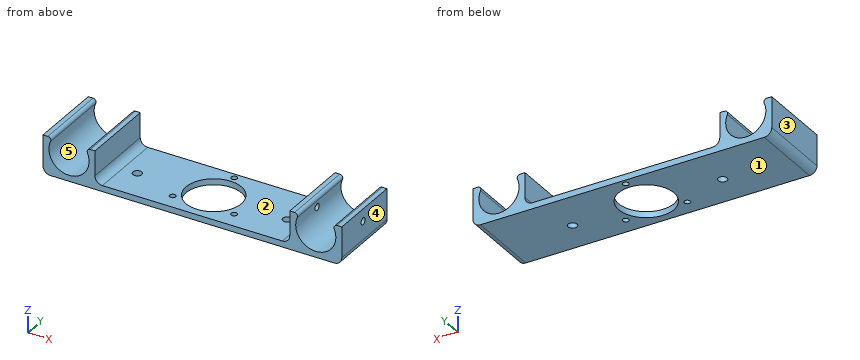
```python
from build123d import *

# Parameters (mm, degrees)
BOSS_EXTRUDE2_START = -1
SKETCH1_R           = 13.45
BOSS_EXTRUDE2_DEPTH = 53
FILLET1_R           = 3
FILLET2_R           = 5
SKETCH9_R           = 2.25
CUT_EXTRUDE2_DEPTH  = 175.062632406
CUT_EXTRUDE4_DEPTH  = 61
FILLET3_R           = 2
SKETCH12_R          = 18.5
SKETCH12_R_2        = 2
CUT_EXTRUDE5_DEPTH  = 61
SKETCH13_R          = 3
CUT_EXTRUDE8_DEPTH  = 41
SKETCH14_W          = 211.811280225
SKETCH14_H          = 13.838629025
CUT_EXTRUDE10_DEPTH = 41


with BuildPart() as part:
    # Sketch1 → Boss-Extrude2 (new body)
    with BuildSketch(Plane(origin=(0, 0, 0), x_dir=(1, 0, 0), z_dir=(0, 1, 0)).offset(BOSS_EXTRUDE2_START)):
        Polygon((-17.4, 17.4), (17.4, 17.4), (17.4, -17.4), (-17.4, -17.4), (-17.4, 13.4), (-82.6, 13.4), (-82.6, 17.4), align=None)
        with Locations(Location((0, 0, 0), (0, 0, 270))):
            Circle(SKETCH1_R, mode=Mode.SUBTRACT)
    boss_extrude2 = extrude(amount=BOSS_EXTRUDE2_DEPTH)

    # Mirror2: Boss-Extrude2 across plane
    add(boss_extrude2.mirror(Plane(origin=(-82.6, -1, -17.4), x_dir=(0, 0, 1), z_dir=(-1, 0, 0))))

    # Fillet1
    fillet1_edges = [part.edges().sort_by_distance(p)[0] for p in [
        (17.4, 25.5, 17.4),
        (-17.4, 25.5, 17.4),
        (-182.6, 25.5, 17.4),
        (-147.8, 25.5, 17.4),
    ]]
    fillet(fillet1_edges, radius=FILLET1_R)

    # Fillet2
    fillet2_edges = [part.edges().sort_by_distance(p)[0] for p in [
        (-17.4, 25.5, -13.4),
        (17.4, 25.5, -17.4),
        (-182.6, 25.5, -17.4),
        (-147.8, 25.5, -13.4),
    ]]
    fillet(fillet2_edges, radius=FILLET2_R)

    # Sketch9 → Cut-Extrude2 (cut, through all)
    with BuildSketch(Plane.ZY.offset(17.4)):
        with Locations((0, 25.5)):
            Circle(SKETCH9_R)
    extrude(amount=-CUT_EXTRUDE2_DEPTH, mode=Mode.SUBTRACT)

    # Sketch11 → Cut-Extrude4 (cut)
    with BuildSketch(Plane.XZ.offset(1)):
        Polygon((17.4, 11.356288415), (17.4, 18.363602968), (-17.4, 18.363602968), (-17.4, 11.356288415), (-17.4, 8.165104504), (-10.6880105, 8.165104504), (10.6880105, 8.165104504), (17.4, 8.165104504), align=None)
        Polygon((-182.6, 11.356288415), (-182.6, 18.363602968), (-147.8, 18.363602968), (-147.8, 11.356288415), (-147.8, 8.165104504), (-154.5119895, 8.165104504), (-175.8880105, 8.165104504), (-182.6, 8.165104504), align=None)
    extrude(amount=-CUT_EXTRUDE4_DEPTH, mode=Mode.SUBTRACT)

    # Fillet3
    fillet3_edges = [part.edges().sort_by_distance(p)[0] for p in [
        (-154.5119895, 25.5, 8.165104504),
        (-175.8880105, 25.5, 8.165104504),
        (10.6880105, 25.5, 8.165104504),
        (-10.6880105, 25.5, 8.165104504),
    ]]
    fillet(fillet3_edges, radius=FILLET3_R)

    # Sketch12 → Cut-Extrude5 (cut)
    with BuildSketch(Plane(origin=(0, 0, -17.4), x_dir=(-1, 0, 0), z_dir=(0, 0, -1))):
        with Locations((82.6, 25.5)):
            Circle(SKETCH12_R)
        with Locations((82.6, 48.25)):
            Circle(SKETCH12_R_2)
        with Locations((102.302077936, 12.625)):
            Circle(SKETCH12_R_2)
        with Locations((61.598883958, 13.375)):
            Circle(SKETCH12_R_2)
    extrude(amount=-CUT_EXTRUDE5_DEPTH, mode=Mode.SUBTRACT)

    # Sketch13 → Cut-Extrude8 (cut)
    with BuildSketch(Plane(origin=(0, 0, -17.4), x_dir=(-1, 0, 0), z_dir=(0, 0, -1))):
        with Locations((132.8, 24)):
            Circle(SKETCH13_R)
        with Locations((32.4, 24)):
            Circle(SKETCH13_R)
    extrude(amount=-CUT_EXTRUDE8_DEPTH, mode=Mode.SUBTRACT)

    # Sketch14 → Cut-Extrude10 (cut)
    with BuildSketch(Plane(origin=(0, 0, -17.4), x_dir=(-1, 0, 0), z_dir=(0, 0, -1))):
        with Locations((80.800037621, -5.103044057)):
            Rectangle(SKETCH14_W, SKETCH14_H)
    extrude(amount=-CUT_EXTRUDE10_DEPTH, mode=Mode.SUBTRACT)


solid = part.part
```
Could you check a few things on this model? Use its own coordinates, in mm. Face numbers are marked on the shaded views. A direction names the side the tool comes from. Coordinates: 2 decimals unless noted, no trailing zeros. Loops run counter-clockwise (first coordinate to the right, second up) from the corner with the lowest first, then second, coordinate; pieces in that order, holes last.
1) Please list where these lines run through material, in increasing order: line 1 along X through (y, z) = (42.5, -10.75); line 2 along X through (y, z) = (21, -1.75); line 3 along Y through (x, z) = (-15.65, 0).
Reported:
line 1: x = -182.6 to -173.28, -157.12 to -147.21, -17.99 to -8.08, 8.08 to 17.4
line 2: x = -182.6 to -178.54, -151.86 to -147.8, -17.4 to -13.34, 13.34 to 17.4
line 3: y = 1.82 to 23.25, 27.75 to 52
2) Thinking about a two-plate mould opening in X: for the marked faces 3, 4 and 5, which applies, released by +X, released by -X, zero draft, split by the parting line, or undercut?
Reported:
face 3: released by -X
face 4: released by +X
face 5: undercut
3) Imagine slicing it at B-B (z = 0). List the corners of the cut face in (x, y) for me.
Reported:
outline: (-182.6, 1.82) - (-178.65, 1.82) - (-178.65, 52) - (-182.6, 52) - close; (-151.75, 1.82) - (-147.8, 1.82) - (-147.8, 52) - (-151.75, 52) - close; (-17.4, 1.82) - (-13.45, 1.82) - (-13.45, 23.25) - (-17.4, 23.25) - close; (-17.4, 27.75) - (-13.45, 27.75) - (-13.45, 52) - (-17.4, 52) - close; (13.45, 1.82) - (17.4, 1.82) - (17.4, 23.25) - (13.45, 23.25) - close; (13.45, 27.75) - (17.4, 27.75) - (17.4, 52) - (13.45, 52) - close
4) Imagine slicing it at C-C (y = 40.5). List the corners of the cut face in (x, z) for me.
Reported:
outline: (-182.6, -12.4) arc R5 ccw to (-177.6, -17.4) - (-93.43, -17.4) - (-93.43, -13.4) - (-142.8, -13.4) arc R5 cw to (-147.8, -8.4) - (-147.8, 8.17) - (-151.03, 8.17) arc R2 ccw to (-152.87, 5.37) arc R13.45 cw (long way) to (-177.53, 5.37) arc R2 ccw to (-179.37, 8.17) - (-182.6, 8.17) - close; (-71.77, -17.4) - (12.4, -17.4) arc R5 ccw to (17.4, -12.4) - (17.4, 8.17) - (14.17, 8.17) arc R2 ccw to (12.33, 5.37) arc R13.45 cw (long way) to (-12.33, 5.37) arc R2 ccw to (-14.17, 8.17) - (-17.4, 8.17) - (-17.4, -8.4) arc R5 cw to (-22.4, -13.4) - (-71.77, -13.4) - close
5) Will these pins go through, and if not, where does the flat tip stop? pin 1 Ø8.5 at (y, z) = (25.5, -1) entering from +X; pin 2 Ø8 at (x, y) = (-133.5, 40) entering from +Z.
Reported:
pin 1: stops at x = 17.4
pin 2: stops at z = -13.4
6) Imagine slicing it at A-A (x = -132.8). List the corners of the cut face in (y, z) for me.
Reported:
outline: (1.82, -17.4) - (21, -17.4) - (21, -13.4) - (1.82, -13.4) - close; (27, -17.4) - (52, -17.4) - (52, -13.4) - (27, -13.4) - close
7) Which directions (+Z, -Z, +X, -X, +Y, -Y) give clear straight access to the entire face, cutting with the end or side of a thin tool? Please do the marked faces 1 and 2.
Reported:
face 1: -Z, +X, -X, +Y, -Y
face 2: +Z, +Y, -Y
8) Imagine slicing it at D-D (x = -71.5). List the corners of the cut face in (y, z) for me.
Reported:
outline: (1.82, -17.4) - (10.7, -17.4) - (10.7, -13.4) - (1.82, -13.4) - close; (40.3, -17.4) - (52, -17.4) - (52, -13.4) - (40.3, -13.4) - close
